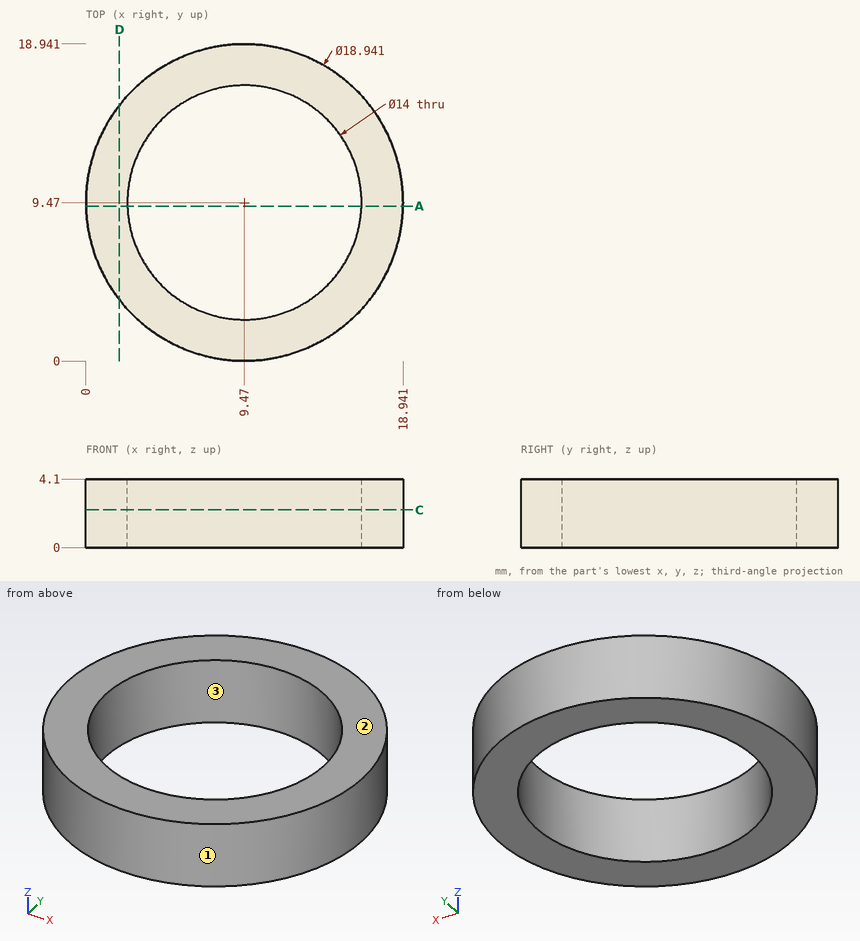
Check sheet for the drawn part. Datum: minimum x, y, z corner. Units: mm. Round coordinates to 2 decimals unless told otherwise and drop trailing zeros. Loops run counter-clockwise (first coordinate to the right, second up) from the corner with the lowest first, then second, coordinate; pieces in that order, holes last. Notation, with made-up numbers: (63, -9) -> (120, -9) arc R9 cw to (120, 1) -> close; hole circle Ø11 at (-11, -39). An arc over 180 degrees is marked (long way). Put each result on its own line as item: value. Start each with the question number.
1. Draft check along Y on the marked faces 1, 2 and 3. Enter one of: +Y half, -Y half, draft (parallel to the pull), parting line (faces both ways), or undercut.
2. Scan lines: probe 1 along X at (y, z) = (9.25, 1.85); probe 2 along X at (y, z) = (10.75, 1.9) (1 decimal); probe 3 along Y at (x, z) = (7.25, 0.4) (1 decimal). Record each from-to range of solid material in increasing order.
3. Gauge pin test, flat ends, axial feed: pin 1 (2 mm diameter, centred on x = 6, z = 0.5, fed in from -Y); pin 2 (11 mm diameter, centred on x = 9.47, y = 9.47, fed in from +Z); pin 3 (1 mm diameter, centred on y = 13, z = 3.5, fed in from -X); pin 4 (2 mm diameter, centred on y = 5.5, z = 3, fed in from +X). Record the tip position at first contact, or that the pin passes through.
4. Section check C-C (z = 2.25). Enter the section's corners in (x, y), plus the area to 3 significant figures.
5. Section check A-A (y = 9.25). Enter the section's corners in (x, z).
6. Section check D-D (x = 2). Enter the section's corners in (y, z).
Findings:
1. face 1: parting line
1. face 2: draft
1. face 3: undercut
2. probe 1: x = 0 to 2.47, 16.47 to 18.94
2. probe 2: x = 0.1 to 2.6, 16.4 to 18.9
2. probe 3: y = 0.3 to 2.8, 16.1 to 18.7
3. pin 1: stops at y = 0.33
3. pin 2: passes through
3. pin 3: stops at x = 0.5
3. pin 4: stops at x = 18.46
4. outline: circle Ø18.94 at (9.47, 9.47); hole circle Ø14 at (9.47, 9.47)
4. area: 128 mm^2
5. outline: (0, 0) -> (2.47, 0) -> (2.47, 4.1) -> (0, 4.1) -> close; (16.47, 0) -> (18.94, 0) -> (18.94, 4.1) -> (16.47, 4.1) -> close
6. outline: (3.65, 0) -> (15.29, 0) -> (15.29, 4.1) -> (3.65, 4.1) -> close
